Input: part model. Units: mm. Frame: model coordinates. Coordinates: 2 decimals unless noted, no trailing zeros. Loops run counter-clockwise (first coordinate to the right, second up) from the corner with the lowest first, then second, coordinate; pieces in that order, holes last.
(1) Section C-C, the plane y = -190.5. Return loops of the section in (x, z), then the cut area to 3 significant figures.
(2) Section B-B, the plane z = 7.75. Give the number of separate pieces and of enclosed holes in the cut face, then the cut area to 3 significant figures.
(3) Section A-A, the plane y = -215.9. Return loops of the section in (x, z).
(4) Section D-D, the plane x = -32.5. Return loops of the section in (y, z), then the cut area to 3 significant figures.
(5) Line query: L1, parallel to Y at x = 37, z = 9.55; L2, parallel to X at y = -215, z = 7.7; L3, parallel to X at y = -239.5, z = 9.95. Output: solid intervals per line, ascending.
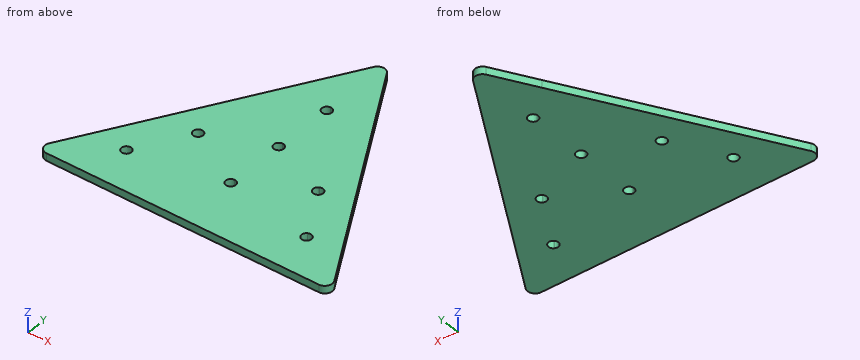
Autodesk Inventor part; units mm, degrees
ref_plane "YZ Plane" through (0, 0, 0) normal (1, 0, 0) x (0, 1, 0)
ref_plane "XZ Plane" through (0, 0, 0) normal (0, 1, 0) x (-1, 0, 0)
ref_plane "XY Plane" through (0, 0, 0) normal (0, 0, 1) x (1, 0, 0)
ref_plane "Work Plane1" through (0, 0, 6.9486) normal (0, 0, 1) x (1, 0, 0)
sketch "Sketch1" plane through (0, 0, 6.9486) normal (0, 0, 1) x (1, 0, 0)
  line L0 (-228.6, -575.3768) -> (0, -179.43)
  line L1 (254, -575.3768) -> (25.4, -179.43)
  line L2 (254, -626.1768) -> (25.4, -230.23)
  arc A0 (51.9003, -250.5775) -> (49.8316, -246.9944) centre (50.8, -248.8241) ccw
  arc A1 (49.6997, -247.0706) -> (51.7684, -250.6537) centre (50.8, -248.8241) ccw
  arc A2 (39.2003, -228.5805) -> (37.1316, -224.9974) centre (38.1, -226.827) ccw
  arc A3 (36.9997, -225.0736) -> (39.0684, -228.6567) centre (38.1, -226.827) ccw
  arc A4 (12.7762, -217.9687) -> (12.7762, -213.8313) centre (12.7, -215.9) ccw
  arc A5 (12.6238, -213.8313) -> (12.6238, -217.9687) centre (12.7, -215.9) ccw
  arc A6 (12.6238, -188.4313) -> (12.6238, -192.5687) centre (12.7, -190.5) ccw
  arc A7 (12.7762, -192.5687) -> (12.7762, -188.4313) centre (12.7, -190.5) ccw
  arc A8 (12.7762, -243.3687) -> (12.7762, -239.2313) centre (12.7, -241.3) ccw
  arc A9 (12.6238, -239.2313) -> (12.6238, -243.3687) centre (12.7, -241.3) ccw
  arc A10 (-26.3684, -250.6537) -> (-24.2997, -247.0706) centre (-25.4, -248.8241) ccw
  arc A11 (-24.4316, -246.9944) -> (-26.5003, -250.5775) centre (-25.4, -248.8241) ccw
  arc A12 (-13.6684, -228.6567) -> (-11.5997, -225.0736) centre (-12.7, -226.827) ccw
  arc A13 (-11.7316, -224.9974) -> (-13.8003, -228.5805) centre (-12.7, -226.827) ccw
  line L3 (12.7, -241.3) -> (12.7, -266.7)
  line L4 (12.7, -266.7) -> (-50.3854, -266.7)
  line L5 (12.7, -266.7) -> (75.7854, -266.7)
  line L6 (75.7854, -266.7) -> (12.7, -157.4329)
  line L7 (-50.3854, -266.7) -> (12.7, -157.4329)
  circle A14 centre (12.7, -190.5) radius 2.0701
  circle A15 centre (12.7, -215.9) radius 2.0701
  circle A16 centre (12.7, -241.3) radius 2.0701
  circle A17 centre (-25.4, -248.8241) radius 2.0701
  circle A18 centre (-12.7, -226.827) radius 2.0701
  circle A19 centre (50.8, -248.8241) radius 2.0701
  circle A20 centre (38.1, -226.827) radius 2.0701
  point P0 (0, 0)
  dimension "d0" = 25.4
extrude "Extrusion1" add sketch "Sketch1" along normal blind 3.175
fillet "Fillet1" radius 3.175 3 edges at (12.7, -157.4329, 8.5361) (-50.3854, -266.7, 8.5361) (75.7854, -266.7, 8.5361)
properties part number "jointplate" material "Aluminum 6061"
Report:
1. outline: (-6.39, 6.95) - (10.63, 6.95) - (10.63, 10.12) - (-6.39, 10.12) - close; (14.77, 6.95) - (31.79, 6.95) - (31.79, 10.12) - (14.77, 10.12) - close
1. area: 108 mm2
2. separate pieces: 1
2. enclosed holes: 7
2. area: 6,780 mm2
3. outline: (-21.06, 6.95) - (10.63, 6.95) - (10.63, 10.12) - (-21.06, 10.12) - close; (14.77, 6.95) - (46.46, 6.95) - (46.46, 10.12) - (14.77, 10.12) - close
4. outline: (-266.7, 6.95) - (-235.72, 6.95) - (-235.72, 10.12) - (-266.7, 10.12) - close
4. area: 98.4 mm2
5. L1: y = -266.7 to -228.58, -225.07 to -199.52
5. L2: x = -20.54 to 10.84, 14.56 to 45.94
5. L3: x = -34.68 to 11.68, 13.72 to 60.08
